Here's how the part is built. I have some questions about the finished solid (model axes, mm). A direction names the side the tool comes from. Coordinates: 2 decimals unless noted, no trailing zeros. Loops run counter-clockwise (first coordinate to the right, second up) from the corner with the lowest first, then second, coordinate; pieces in that order, holes last. Notation, with made-up numbers: (18.25, 86.25) -> (45.25, 86.25) arc R24 cw to (45.25, 116.25) -> close; hole circle Ø4 at (12.5, 26.25). An arc over 180 degrees is marked (long way). Answer as a JSON object with one key per item and string values. Group by question number.
Q1. I want a section at D-D on z = -1. Write out the boundary of the cut face in (x, y).
Q2. I want a section at C-C on x = -22.5. Write out the boundary of the cut face in (y, z), then the cut area to 3 significant figures.
Q3. I need wall thicknesses on line 1 (Y direction, x = 18, z = -23). Which ranges of the line are inside material? Lowest first, please.
Q4. I want a section at A-A on y = 14.5. Write out the boundary of the cut face in (x, z) (3 decimals), then the cut area to 3 significant figures.
Q5. Thinking about a two-plate mould opening in Z: for faces 6 (the flat face through (-43, 17.5, 13)), 7 (the flat face through (-43, 14, -10.795)), 8 (the flat face through (-43, 14, -14.605)), which applies, released by +Z, released by -Z, zero draft, split by the parting line, or undercut?
Q6. On a 3-axis mill with a long thin cutter (end or side, diameter ignored), from which of +Z, -Z, +X, -X, +Y, -Y can I reach the whole of each face in a straight line? I mean faces 1 (the flat face through (-1, 0, 0)), 2 (the flat face through (40, 14, -13)), 3 (the flat face through (43, 14, -14.605)), 4 (the flat face through (43, 14, 14.605)), 5 (the flat face through (43, 14, 10.795)). Say none if no direction works.
Q7. I'm going to push flat-ended pins straight in: pin 1 (1.5 mm diameter, centred on x = 43.5, y = 15.5, fed in from -Z) (3 decimals); pin 2 (2.5 mm diameter, centred on x = 41.5, y = 15, fed in from +Z) (3 decimals). Where does each tip first touch, or does it pass through?
Q8. I want a section at B-B on z = -12. Write out the boundary of the cut face in (x, y).
```python
from build123d import *

# Parameters (mm, degrees)
SKETCH1_W           = 90
SKETCH1_H           = 60
BOSS_EXTRUDE1_DEPTH = 10
SKETCH4_W           = 3.81
SKETCH4_H           = 7.5
BOSS_EXTRUDE2_DEPTH = 5


with BuildPart() as part:
    # Sketch1 → Boss-Extrude1 (new body)
    with BuildSketch(Plane(origin=(0, 0, 0), x_dir=(1, 0, 0), z_dir=(0, 1, 0))):
        Rectangle(SKETCH1_W, SKETCH1_H)
    extrude(amount=BOSS_EXTRUDE1_DEPTH)

    # Sketch4 → Boss-Extrude2 (add)
    with BuildSketch(Plane.ZY.offset(45)):
        with Locations((-12.7, 13.75)):
            Rectangle(SKETCH4_W, SKETCH4_H)
        with Locations((12.7, 13.75)):
            Rectangle(SKETCH4_W, SKETCH4_H)
    boss_extrude2 = extrude(amount=-BOSS_EXTRUDE2_DEPTH)

    # Mirror1: Boss-Extrude2 across plane
    add(boss_extrude2.mirror(Plane(origin=(0, 0, 0), x_dir=(0, 0, 1), z_dir=(1, 0, 0))))


solid = part.part
```
Result set:
{
 "1": {"outline": "(-45, 0) -> (45, 0) -> (45, 10) -> (-45, 10) -> close"},
 "2": {"outline": "(0, -30) -> (10, -30) -> (10, 30) -> (0, 30) -> close", "area": "600 mm²"},
 "3": {"line 1": "y = 0 to 10"},
 "4": {"outline": "(-45, -14.605) -> (-40, -14.605) -> (-40, -10.795) -> (-45, -10.795) -> close; (-45, 10.795) -> (-40, 10.795) -> (-40, 14.605) -> (-45, 14.605) -> close; (40, -14.605) -> (45, -14.605) -> (45, -10.795) -> (40, -10.795) -> close; (40, 10.795) -> (45, 10.795) -> (45, 14.605) -> (40, 14.605) -> close", "area": "76.2 mm²"},
 "5": {"face 6": "zero draft", "face 7": "undercut", "face 8": "released by -Z"},
 "6": {"face 1": "+Z, -Z, +X, -X, -Y", "face 2": "+Z, -Z, +Y", "face 3": "-Z, +X, -X, +Y", "face 4": "+Z, +X, -X, +Y", "face 5": "+X, -X, +Y"},
 "7": {"pin 1": "stops at z = -14.605", "pin 2": "stops at z = 14.605"},
 "8": {"outline": "(-45, 0) -> (45, 0) -> (45, 17.5) -> (40, 17.5) -> (40, 10) -> (-40, 10) -> (-40, 17.5) -> (-45, 17.5) -> close"}
}
